Check sheet for the drawn part. Datum: minimum x, y, z corner. Units: mm. A direction names the side the tool comes from. Coordinates: 2 decimals unless noted, no trailing zeros. Order: outer loops, then holes, each group sorted by start corner. A loop starts at its lowest first (then second) coordinate and runs counter-clockwise, first axis right, second up.
1. Cross-section at B-B (x = 14.25). Enter the section's corners in (y, z).
2. Set-up check for the marked faces 4 and 5: record each of +Z, -Z, +X, -X, +Y, -Y from which the full face is reachable in a straight line by a thin tool's end or side.
3. Draft check along Y on the marked faces 1, 2 and 3. Enter one of: released by +Y, released by -Y, zero draft, split by the parting line, or undercut.
4. Cross-section at A-A (z = 2). Count the separate pieces of the cut face and the enclosed holes in it.
5. Cross-section at D-D (y = 11.5). Enter the section's corners in (x, z) (1 decimal).
6. Gauge pin test, flat ends, axial feed: pin 1 Ø3 at (x, y) = (11.62, 3.12) entering from +Z; pin 2 Ø1.9 at (x, y) = (2.286, 8.509) entering from -Z; pin 3 Ø1.6 at (y, z) = (9, 2) entering from +X; pin 4 Ø2 at (y, z) = (3.5, 3.5) entering from +X (1 decimal). Record the tip position at first contact, or that the pin passes through.
7. Thickness scan on line 1 (X direction, y = 8.5, z = 1.15) (1 decimal); line 2 (Y direction, x = 8.5, z = 1.5); line 3 (X direction, y = 13.5, z = 3.2). Record the ranges inside material, lowest first.
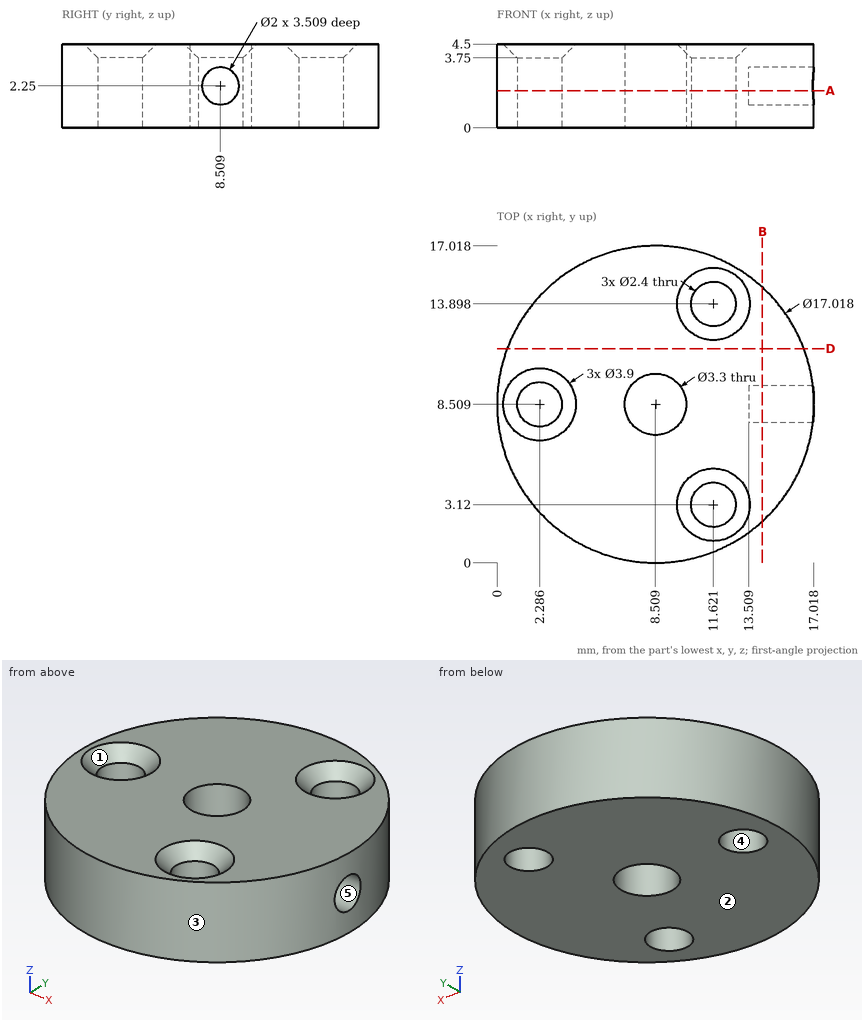
Data:
1. outline: (2.23, 0) - (14.79, 0) - (14.79, 4.5) - (2.23, 4.5) - close; hole circle Ø2 at (8.51, 2.25)
2. face 4: +Z, -Z
2. face 5: +X
3. face 1: undercut
3. face 2: zero draft
3. face 3: split by the parting line
4. separate pieces: 1
4. enclosed holes: 4
5. outline: (0.5, 0) - (16.5, 0) - (16.5, 4.5) - (0.5, 4.5) - close
6. pin 1: stops at z = 4.05
6. pin 2: passes through
6. pin 3: stops at x = 17.02
6. pin 4: stops at x = 16
7. line 1: x = 0 to 1.1, 3.5 to 6.9, 10.2 to 17
7. line 2: y = 0 to 6.86, 10.16 to 17.02
7. line 3: x = 1.62 to 10.49, 12.75 to 15.4
